Here's how the part is built. I have some questions about the finished solid (model axes, mm). Round coordinates to 2 decimals unless told otherwise and drop trailing zeros. Loops run counter-clockwise (first coordinate to the right, second up) from the corner with the lowest first, then second, coordinate; pieces in that order, holes last. Notation, with made-up numbers: (43, -33.75) - (62, -33.75) arc R12 cw to (62, -14.75) - close; hole circle Ø3 at (61.5, 22). An arc over 180 degrees is marked (long way). Answer as a JSON object with one key per item and string values. Group by question number.
1) If I drill on line 1 along Y through (x, z) = (-1.35, 0); line 2 along Z through (x, y) = (-1.75, 167.5); line 3 along Z through (x, y) = (1, 538), over which ranges is the centre line in solid material (lowest first)? Write a range as [from, to].
2) Will these pins go through, and if not, where does the flat tip stop? P1, Ø5, axis at x = -1.5, y = 473.5, coming from the +Z side; P2, Ø1, axis at x = -3.5, z = -15.5, coming from the -Y side; P3, Ø1.5, axis at x = -1, z = 98, coming from the +Y side.
3) I want a section at A-A, the plane y = 204.5. Please give me the cut outline in (x, z).
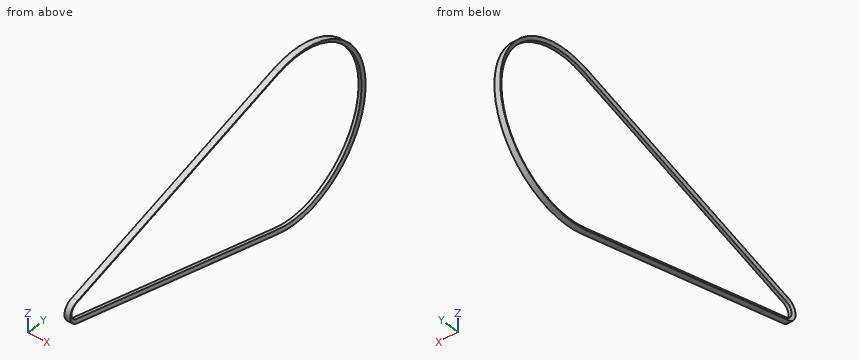
from build123d import *


with BuildPart() as f2:
    # F2: sweep along a path in F0
    with BuildLine(Plane.YZ) as f2_path:
        ThreePointArc((411.7521428571, -128.3438525018), (581.2971428571, 0), (411.7521428571, 128.3438525018))
        Line((411.7521428571, 128.3438525018), (0, 12.2232240478))
        ThreePointArc((0, 12.2232240478), (-9.2528571429, 0), (0, -12.2232240478))
        Line((0, -12.2232240478), (411.7521428571, -128.3438525018))
    # F1 (on Front) → F2 (sweep)
    with BuildSketch(Plane.XZ):
        Polygon((-4.7625, 18.7229695863), (-2.468474675, 13.1667195863), (2.468474675, 13.1667195863), (4.7625, 18.7229695863), align=None)
    sweep(path=f2_path.line)


solid = f2.part
Outcome:
{
 "1": {"line 1": "[-15.59, -10.16], [582.21, 587.56]", "line 2": "[-65.96, -60.4], [60.4, 65.96]", "line 3": "[-106.69, -99.58], [99.58, 106.69]"},
 "2": {"P1": "z = 137.7", "P2": "y = -8.28", "P3": "y = 548.12"},
 "3": {"outline": "(-4.76, -76.4) - (4.76, -76.4) - (2.47, -70.84) - (-2.47, -70.84) - close; (-4.76, 76.4) - (-2.47, 70.84) - (2.47, 70.84) - (4.76, 76.4) - close"}
}
